from build123d import *

# Parameters (mm, degrees)
CHAMFER1_SIZE       = 10
SKETCH2_R           = 1.25
CUT_EXTRUDE1_DEPTH  = 30
SKETCH5_R           = 5.5
BOSS_EXTRUDE1_DEPTH = 62.5
SKETCH3_R           = 35
CUT_EXTRUDE2_DEPTH  = 25
SKETCH4_R           = 20
CUT_EXTRUDE3_DEPTH  = 32
FILLET1_R           = 5
FILLET2_R           = 3
SKETCH6_R           = 3
CUT_EXTRUDE4_DEPTH  = 146.151644955


with BuildPart() as part:
    # Sketch1 → Revolve1 (revolve)
    with BuildSketch(Plane(origin=(0, 0, 0), x_dir=(1, 0, 0), z_dir=(0, 1, 0)), mode=Mode.PRIVATE) as revolve1_sk:
        Polygon((0, 0), (40, 0), (40, 35), (25.5, 35), (25.5, 62), (0, 62), align=None)
    revolve(revolve1_sk.sketch.rotate(Axis((0, 0, -62), (0, 0, 1)), 180), axis=Axis((0, 0, -62), (0, 0, 1)))

    # Chamfer1
    chamfer1_edges = [part.edges().sort_by_distance(p)[0] for p in [
        (25.5, 0, -35),
    ]]
    chamfer(chamfer1_edges, length=CHAMFER1_SIZE)

    # Sketch2 → Cut-Extrude1 (cut)
    with BuildSketch(Plane(origin=(0, 0, -62), x_dir=(-1, 0, 0), z_dir=(0, 0, -1))):
        Circle(SKETCH2_R)
    extrude(amount=-CUT_EXTRUDE1_DEPTH, mode=Mode.SUBTRACT)

    # Sketch5 → Boss-Extrude1 (add, symmetric)
    with BuildSketch(Plane(origin=(0, 0, 0), x_dir=(1, 0, 0), z_dir=(0, 1, 0))):
        with Locations(Location((0, 10, 0), (0, 0, 90))):
            Circle(SKETCH5_R)
    extrude(amount=BOSS_EXTRUDE1_DEPTH, both=True)

    # Sketch3 → Cut-Extrude2 (cut)
    with BuildSketch(Plane.XY):
        Circle(SKETCH3_R)
    extrude(amount=-CUT_EXTRUDE2_DEPTH, mode=Mode.SUBTRACT)

    # Sketch4 → Cut-Extrude3 (cut)
    with BuildSketch(Plane.XY.offset(-25)):
        Circle(SKETCH4_R)
    extrude(amount=-CUT_EXTRUDE3_DEPTH, mode=Mode.SUBTRACT)

    # Fillet1
    fillet1_edges = [part.edges().sort_by_distance(p)[0] for p in [
        (-35, 0, -25),
        (-20, 0, -57),
        (-20, 0, -25),
    ]]
    fillet(fillet1_edges, radius=FILLET1_R)

    # Fillet2
    fillet2_edges = [part.edges().sort_by_distance(p)[0] for p in [
        (0, -40, -4.5),
        (0, 40, -4.5),
    ]]
    fillet(fillet2_edges, radius=FILLET2_R)

    # Sketch6 → Cut-Extrude4 (cut, through all)
    with BuildSketch(Plane(origin=(0, 62.5, 0), x_dir=(1, 0, 0), z_dir=(0, 1, 0))):
        with Locations(Location((0, 10, 0), (0, 0, 270))):
            Circle(SKETCH6_R)
    extrude(amount=-CUT_EXTRUDE4_DEPTH, mode=Mode.SUBTRACT)


solid = part.part
Input: part model. Units: mm. Frame: model coordinates. A direction names the side the tool comes from. Coordinates: 2 decimals unless noted, no trailing zeros. Order: outer loops, then holes, each group sorted by start corner. A loop starts at its lowest first (then second) coordinate and runs counter-clockwise, first axis right, second up. Notation, with made-up numbers: M 3.5,83.25 L 22.5,83.25 A25 cw 22.5,119.25 Z; hole C -24,21.5 d3. An arc over 180 degrees is marked long. Write item = value, one per line. Start each with the question number.
(1) First-contact query: P1, Ø1.5, axis at y = -35, z = -21, coming from the +X side; P2, Ø3, axis at y = 18, z = -54, coming from the -X side; P3, Ø5, axis at x = -31.5, z = -31.5, coming from the +Y side; P4, Ø7, axis at x = 0, z = -10, coming from the +Y side. Flat tips, straight axial feed; report the tip coordinate or a pass-through.
(2) Reachability of faces 4 (the cylindrical face through (2.11, 52.47, -15.08)), 5 (the cylindrical face through (5.5, 24.9, -53.6)), 6 (the cylindrical face through (2.11, -52.18, -15.08)), 7 (the flat face through (2.4, 62.5, -12.4)), 8 (the cylindrical face through (-4.336, -19.524, -40.846)) from +Z, -Z, +X, -X, +Y, -Y: full face, straight path, thin tool, end or side. Return the list, or none.
(3) Pull-direction query (Z, two-part tool) for faces 1 (the cylindrical face through (0, 49, -13)), 2 (the flat face through (0, -3, -57)), 3 (the flat face through (2.4, -62.5, -12.4)); classes: released by +Z, released by -Z, zero draft, split by the parting line, or undercut.
(4) Line query: line 1 along Y through (x, z) = (0, -59); line 2 along Y through (x, z) = (0, -5); line 3 along X through (y, z) = (-55, -10). Output: solid intervals per line, ascending. Write a range as [from, to].
(5) Section A-A on z = -37.5. Output: boundary loops of the cut face in (x, y), and give its area (3 significant figures).
(6) Section B-B on y = 53.5. Output: boundary loops of the cut face in (x, z).
Result set:
q1.P1 = 20.66
q1.P2 = -19.44
q1.P3 = 27.55
q1.P4 = 62.5
q2.face_4 = +Y
q2.face_5 = -Z
q2.face_6 = -Y
q2.face_7 = +Z, -Z, +X, -X, +Y
q2.face_8 = +Z
q3.face_1 = undercut
q3.face_2 = released by +Z
q3.face_3 = zero draft
q4.line_1 = [-25.5, -1.25], [1.25, 25.5]
q4.line_2 = [-62.5, -35], [35, 62.5]
q4.line_3 = [-5.5, -3], [3, 5.5]
q5.outline = C 0,0 d66; hole C 0,0 d40
q5.area = 2,160 mm²
q6.outline = C 0,-10 d11; hole C 0,-10 d6
